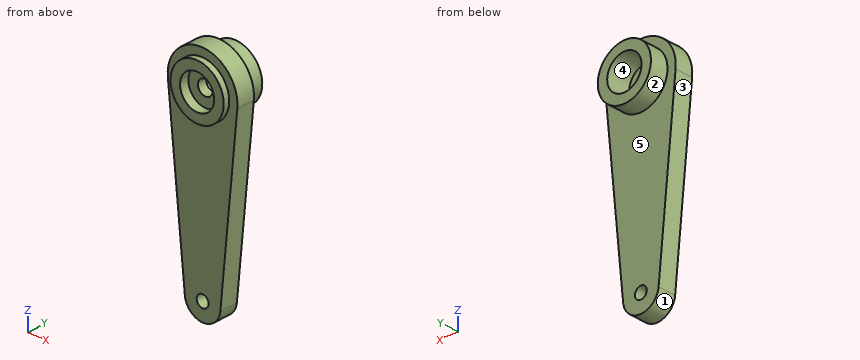
from build123d import *

# Parameters (mm, degrees)
SKETCH2_R           = 1
SKETCH2_R_2         = 2.9
BOSS_EXTRUDE1_DEPTH = 3
SKETCH2_4_R         = 2.9
SKETCH2_4_R_2       = 1.25
BOSS_EXTRUDE2_DEPTH = 2
SKETCH7_R           = 4.5
SKETCH7_R_2         = 2.9
BOSS_EXTRUDE3_DEPTH = 3
BOSS_EXTRUDE4_START = 1
SKETCH8_R           = 4.5
SKETCH8_R_2         = 2.875
BOSS_EXTRUDE4_DEPTH = 1
SKETCH9_R           = 2.875
CUT_EXTRUDE2_DEPTH  = 0.5


with BuildPart() as part:
    # Sketch2 → Boss-Extrude1 (new body)
    with BuildSketch(Plane(origin=(0, 0, 0), x_dir=(1, 0, 0), z_dir=(0, 1, 0))):
        with BuildLine():
            Line((-3, 30.28994689), (-5.872635545, 0.567584137))
            ThreePointArc((-5.872635545, 0.567584137), (0, -5.9), (5.872635545, 0.567584137))
            Line((5.872635545, 0.567584137), (3, 30.28994689))
            ThreePointArc((3, 30.28994689), (0, 33.013978965), (-3, 30.28994689))
        make_face()
        with Locations(Location((0, 30, 0), (0, 0, 270))):
            Circle(SKETCH2_R, mode=Mode.SUBTRACT)
        with Locations(Location((0, 0, 0), (0, 0, 270))):
            Circle(SKETCH2_R_2, mode=Mode.SUBTRACT)
    extrude(amount=BOSS_EXTRUDE1_DEPTH)

    # Sketch2_4 → Boss-Extrude2 (add)
    with BuildSketch(Plane(origin=(0, 0, 0), x_dir=(1, 0, 0), z_dir=(0, 1, 0))):
        with Locations(Location((0, 0, 0), (0, 0, 270))):
            Circle(SKETCH2_4_R)
        with Locations(Location((0, 0, 0), (0, 0, 270))):
            Circle(SKETCH2_4_R_2, mode=Mode.SUBTRACT)
    extrude(amount=BOSS_EXTRUDE2_DEPTH)

    # Sketch7 → Boss-Extrude3 (add)
    with BuildSketch(Plane(origin=(0, 3, 0), x_dir=(1, 0, 0), z_dir=(0, 1, 0))):
        with Locations(Location((0, 0, 0), (0, 0, 270))):
            Circle(SKETCH7_R)
        with Locations(Location((0, 0, 0), (0, 0, 270))):
            Circle(SKETCH7_R_2, mode=Mode.SUBTRACT)
    extrude(amount=BOSS_EXTRUDE3_DEPTH)

    # Sketch8 → Boss-Extrude4 (add)
    with BuildSketch(Plane.XZ.offset(BOSS_EXTRUDE4_START)):
        with Locations(Location((0, 0, 0), (0, 0, 90))):
            Circle(SKETCH8_R)
        with Locations(Location((0, 0, 0), (0, 0, 270))):
            Circle(SKETCH8_R_2, mode=Mode.SUBTRACT)
    extrude(amount=-BOSS_EXTRUDE4_DEPTH)

    # Sketch9 → Cut-Extrude2 (cut)
    with BuildSketch(Plane.XZ):
        with Locations(Location((0, 0, 0), (0, 0, 270))):
            Circle(SKETCH9_R)
    extrude(amount=-CUT_EXTRUDE2_DEPTH, mode=Mode.SUBTRACT)


solid = part.part
Design review of the part built by this model. Coordinates are the model's own, in mm. Face numbers are marked on the shaded views. A direction names the side the tool comes from. Coordinates: 2 decimals unless noted, no trailing zeros. Order: outer loops, then holes, each group sorted by start corner. A loop starts at its lowest first (then second) coordinate and runs counter-clockwise, first axis right, second up. Notation, with made-up numbers: M 49.25,66 L 97.25,66 A9 ccw 97.25,77 Z; hole C 43.25,61 d3. An arc over 180 degrees is marked long. Use a Markdown table: item, result.
(1) Draft analysis for pull direction Z (two halves, no side actions). For the marked faces 3, 4 and 5, state which applies: released by +Z, released by -Z, zero draft, split by the parting line, or undercut.
Worked answers:
| item | result |
|---|---|
| face 3 | released by -Z |
| face 4 | undercut |
| face 5 | zero draft |
(2) For P1, Ø3, axis at x = 0, z = -30, coming from the -Y side; P2, Ø4, axis at x = 4, z = -15.5, coming from the +Y side; P3, Ø3, axis at y = 5, z = 1.5, coming from the -X side; P4, Ø3, axis at y = 5, z = -8.5, coming from the -X side, all flat-tipped, find the tip position at first contact; note any pin that passes through.
Worked answers:
| item | result |
|---|---|
| P1 | stops at y = 0 |
| P2 | stops at y = 3 |
| P3 | stops at x = -4.5 |
| P4 | passes through |
(3) Add section D-D (x = 4). Give the boundary of the cut face in (y, z).
Worked answers:
| item | result |
|---|---|
| outline | M -1,-2.06 L 0,-2.06 L 0,-19.94 L 3,-19.94 L 3,-2.06 L 6,-2.06 L 6,2.06 L 3,2.06 L 3,4.34 L 0,4.34 L 0,2.06 L -1,2.06 Z |
(4) Add section A-A (z = 0). Give the boundary of the cut face in (x, y) (3 decimals).
Worked answers:
| item | result |
|---|---|
| outline | M -5.9,0 L -4.5,0 L -4.5,-1 L -2.875,-1 L -2.875,0.5 L -1.25,0.5 L -1.25,2 L -2.9,2 L -2.9,6 L -4.5,6 L -4.5,3 L -5.9,3 Z; M 1.25,0.5 L 2.875,0.5 L 2.875,-1 L 4.5,-1 L 4.5,0 L 5.9,0 L 5.9,3 L 4.5,3 L 4.5,6 L 2.9,6 L 2.9,2 L 1.25,2 Z |
(5) Add section C-C (y = 1.25). Give the boundary of the cut face in (x, z).
Worked answers:
| item | result |
|---|---|
| outline | M -5.87,-0.57 L -3,-30.29 A3.01 ccw 3,-30.29 L 5.87,-0.57 A5.9 ccw long Z; hole C 0,0 d2.5; hole C 0,-30 d2 |
(6) Add section B-B (x = 0). Give the boundary of the cut face in (y, z) (3 decimals), then the cut area to 3 significant figures.
Worked answers:
| item | result |
|---|---|
| outline | M -1,-4.5 L 0,-4.5 L 0,-29 L 3,-29 L 3,-4.5 L 6,-4.5 L 6,-2.9 L 2,-2.9 L 2,-1.25 L 0.5,-1.25 L 0.5,-2.875 L -1,-2.875 Z; M -1,2.875 L 0.5,2.875 L 0.5,1.25 L 2,1.25 L 2,2.9 L 6,2.9 L 6,4.5 L 3,4.5 L 3,5.9 L 0,5.9 L 0,4.5 L -1,4.5 Z; M 0,-33.014 L 3,-33.014 L 3,-31 L 0,-31 Z |
| area | 111 mm2 |
(7) Wall thickness on probe 1 along Y at (x, z) = (-3.25, -25.5); probe 2 along X at (y, z) = (1.65, 0); probe 3 along X at (y, z) = (-0.25, 0) (3 decimals): over which ranges is each line inside the solid? List them lowest first.
Worked answers:
| item | result |
|---|---|
| probe 1 | y = 0 to 3 |
| probe 2 | x = -5.9 to -1.25, 1.25 to 5.9 |
| probe 3 | x = -4.5 to -2.875, 2.875 to 4.5 |
(8) For the marked faces 1 and 2, list the 3-axis set-ups (+Z, -Z, +X, -X, +Y, -Y) from which the entire face can be reached by the end or side of a thin tool; tool diameter is ignored.
Worked answers:
| item | result |
|---|---|
| face 1 | -Z, +Y, -Y |
| face 2 | +Y |
